```python
from build123d import *

# Parameters (mm, degrees)
CROQUIS1_W                         = 730
CROQUIS1_H                         = 400
BRIDA_BASE1_DEPTH                  = 2.9
BRIDA_DE_ARISTA1_STRIP_W           = 13.0732
BRIDA_DE_ARISTA1_STRIP_H           = 2.9
BRIDA_DE_ARISTA1_STRIP_CUT_DEPTH   = 730
BRIDA_DE_ARISTA1_STRIP_2_W         = 13.0732
BRIDA_DE_ARISTA1_STRIP_2_H         = 2.9
BRIDA_DE_ARISTA1_STRIP_CUT_2_DEPTH = 730
BRIDA_DE_ARISTA1_DEPTH             = 730
BRIDA_DE_ARISTA1_BEND_DEPTH        = 730
BRIDA_DE_ARISTA2_STRIP_W           = 13.0732
BRIDA_DE_ARISTA2_STRIP_H           = 2.9
BRIDA_DE_ARISTA2_STRIP_CUT_DEPTH   = 730
BRIDA_DE_ARISTA2_STRIP_2_W         = 13.0732
BRIDA_DE_ARISTA2_STRIP_2_H         = 2.9
BRIDA_DE_ARISTA2_STRIP_CUT_2_DEPTH = 730
BRIDA_DE_ARISTA2_DEPTH             = 730
BRIDA_DE_ARISTA2_BEND_DEPTH        = 730
CROQUIS18_W                        = 653.8
CROQUIS18_H                        = 36.3634
CORTAR_EXTRUIR1_DEPTH              = 4


# Sheet-metal steps are written as plain solids
with BuildPart() as part:
    # Croquis1 → Brida base1 (new body)
    with BuildSketch(Plane(origin=(0, 0, 0), x_dir=(1, 0, 0), z_dir=(0, 1, 0))):
        Rectangle(CROQUIS1_W, CROQUIS1_H)
    extrude(amount=-BRIDA_BASE1_DEPTH)

    # Brida de arista1 strip (across the edge) → Brida de arista1 strip cut (cut)
    with BuildSketch(Plane(origin=(365, 0, -200), x_dir=(0, 0, 1), z_dir=(-1, 0, 0))):
        with Locations((-2.9, -1.45)):
            Rectangle(BRIDA_DE_ARISTA1_STRIP_W, BRIDA_DE_ARISTA1_STRIP_H)
    extrude(amount=BRIDA_DE_ARISTA1_STRIP_CUT_DEPTH, mode=Mode.SUBTRACT)

    # Brida de arista1 strip 2 (across the edge) → Brida de arista1 strip cut 2 (cut)
    with BuildSketch(Plane(origin=(-365, 0, 200), x_dir=(0, 0, -1), z_dir=(1, 0, 0))):
        with Locations((-2.9, -1.45)):
            Rectangle(BRIDA_DE_ARISTA1_STRIP_2_W, BRIDA_DE_ARISTA1_STRIP_2_H)
    extrude(amount=BRIDA_DE_ARISTA1_STRIP_CUT_2_DEPTH, mode=Mode.SUBTRACT)

    # Brida de arista1 section (across the edge) → Brida de arista1 (add)
    with BuildSketch(Plane(origin=(365, 0, -200), x_dir=(0, 0, 1), z_dir=(-1, 0, 0))):
        with BuildLine():
            Line((0, 0.7366), (0, 272.1))
            Line((0, 272.1), (2.9, 272.1))
            Line((2.9, 272.1), (2.9, 0.7366))
            ThreePointArc((2.9, 0.7366), (3.115745145, 0.215745145), (3.6366, 0))
            Line((3.6366, 0), (3.6366, -2.9))
            ThreePointArc((3.6366, -2.9), (1.06513548, -1.83486452), (0, 0.7366))
        make_face()
    extrude(amount=BRIDA_DE_ARISTA1_DEPTH)

    # Brida de arista1 section 2 (across the edge) → Brida de arista1 bend (add)
    with BuildSketch(Plane(origin=(-365, 0, 200), x_dir=(0, 0, -1), z_dir=(1, 0, 0))):
        with BuildLine():
            Line((0, 0.7366), (0, 272.1))
            Line((0, 272.1), (2.9, 272.1))
            Line((2.9, 272.1), (2.9, 0.7366))
            ThreePointArc((2.9, 0.7366), (3.115745145, 0.215745145), (3.6366, 0))
            Line((3.6366, 0), (3.6366, -2.9))
            ThreePointArc((3.6366, -2.9), (1.06513548, -1.83486452), (0, 0.7366))
        make_face()
    extrude(amount=BRIDA_DE_ARISTA1_BEND_DEPTH)

    # Brida de arista2 strip (across the edge) → Brida de arista2 strip cut (cut)
    with BuildSketch(Plane(origin=(365, 272.1, -197.1), x_dir=(0, -1, 0), z_dir=(-1, 0, 0))):
        with Locations((-2.9, -1.45)):
            Rectangle(BRIDA_DE_ARISTA2_STRIP_W, BRIDA_DE_ARISTA2_STRIP_H)
    extrude(amount=BRIDA_DE_ARISTA2_STRIP_CUT_DEPTH, mode=Mode.SUBTRACT)

    # Brida de arista2 strip 2 (across the edge) → Brida de arista2 strip cut 2 (cut)
    with BuildSketch(Plane(origin=(-365, 272.1, 197.1), x_dir=(0, -1, 0), z_dir=(1, 0, 0))):
        with Locations((-2.9, -1.45)):
            Rectangle(BRIDA_DE_ARISTA2_STRIP_2_W, BRIDA_DE_ARISTA2_STRIP_2_H)
    extrude(amount=BRIDA_DE_ARISTA2_STRIP_CUT_2_DEPTH, mode=Mode.SUBTRACT)

    # Brida de arista2 section (across the edge) → Brida de arista2 (add)
    with BuildSketch(Plane(origin=(365, 272.1, -197.1), x_dir=(0, -1, 0), z_dir=(-1, 0, 0))):
        with BuildLine():
            Line((0, 0.7366), (0, 37.1))
            Line((0, 37.1), (2.9, 37.1))
            Line((2.9, 37.1), (2.9, 0.7366))
            ThreePointArc((2.9, 0.7366), (3.115745145, 0.215745145), (3.6366, 0))
            Line((3.6366, 0), (3.6366, -2.9))
            ThreePointArc((3.6366, -2.9), (1.06513548, -1.83486452), (0, 0.7366))
        make_face()
    extrude(amount=BRIDA_DE_ARISTA2_DEPTH)

    # Brida de arista2 section 2 (across the edge) → Brida de arista2 bend (add)
    with BuildSketch(Plane(origin=(-365, 272.1, 197.1), x_dir=(0, -1, 0), z_dir=(1, 0, 0))):
        with BuildLine():
            Line((0, 0.7366), (0, 37.1))
            Line((0, 37.1), (2.9, 37.1))
            Line((2.9, 37.1), (2.9, 0.7366))
            ThreePointArc((2.9, 0.7366), (3.115745145, 0.215745145), (3.6366, 0))
            Line((3.6366, 0), (3.6366, -2.9))
            ThreePointArc((3.6366, -2.9), (1.06513548, -1.83486452), (0, 0.7366))
        make_face()
    extrude(amount=BRIDA_DE_ARISTA2_BEND_DEPTH)

    # Croquis18 → Cortar-Extruir1 (cut)
    with BuildSketch(Plane(origin=(0, 272.1, 0), x_dir=(1, 0, 0), z_dir=(0, 1, 0))):
        with Locations((0, -178.1817)):
            Rectangle(CROQUIS18_W, CROQUIS18_H)
        with Locations((0, 178.1817)):
            Rectangle(CROQUIS18_W, CROQUIS18_H)
    extrude(amount=-CORTAR_EXTRUIR1_DEPTH, mode=Mode.SUBTRACT)


solid = part.part
```
CAD build for the part. Positions are in the model's coordinates, mm. A direction names the side the tool comes from. Coordinates: 2 decimals unless noted, no trailing zeros. Write each loop counter-clockwise with the first axis right and the second up, starting at its lowest first coordinate (ties: lowest second). Pieces come first, ordered by that corner, then holes. Notation, with made-up numbers: (-38.75, 87.25) -> (-34.75, 87.25) arc R36 ccw to (-34.75, 123.25) -> close; hole circle Ø2 at (10, 26). An arc over 180 degrees is marked (long way). Return JSON: item names as keys, results as strings. Group by question number.
Q1. Drill centre lines: line 1 (Z direction, x = -223.5, y = 226.5); line 2 (Y direction, x = 2, z = 19). Where is each one in solid material? Low to high.
Q2. Flat gauge pins, fed straight in: pin 1 (2.5 mm diameter, centred on x = 346, y = 270.5, fed in from -Z); pin 2 (3 mm diameter, centred on x = -353, y = 271, fed in from -Z); pin 3 (0.9 mm diameter, centred on x = -336.5, y = 270.5, fed in from +Z). Where does each tip first touch, or does it go through?
Q3. Cut at B-B, the plane x = -58. Give the cut face in (y, z), then the cut area to 3 significant figures.
Q4. Pull direction Y, two halves, no side cores. Call faces 3 (the face through (-5, -2.9, -3)), 4 (the face through (-346, 272.1, 178)), 5 (the face through (5, 136, -197.1)), 6 (the face through (-346, 269.2, -178)): released by +Y, released by -Y, zero draft, split by the parting line, or undercut.
Q5. Cut at A-A, the plane y = 208. Give the cut face in (x, z).
Q6. Cut at C-C, the plane z = -49.5. Give the cut face in (x, y).
Q7. Which spindle directions (+Z, -Z, +X, -X, +Y, -Y) get a long thin tool onto all of the face, cutting with end or side? Do faces 1 (the face through (346, 272.1, -178)), 2 (the face through (346, 269.2, -178)). Say none if no direction does.
Returned:
{
 "1": {"line 1": "z = -200 to -197.1, 197.1 to 200", "line 2": "y = -2.9 to 0"},
 "2": {"pin 1": "stops at z = -199.91", "pin 2": "stops at z = -199.85", "pin 3": "stops at z = 199.64"},
 "3": {"outline": "(-2.9, -196.36) arc R3.64 ccw to (0.74, -200) -> (268.46, -200) arc R3.64 ccw to (272.1, -196.36) -> (269.2, -196.36) arc R0.74 cw to (268.46, -197.1) -> (0.74, -197.1) arc R0.74 cw to (0, -196.36) -> (0, 196.36) arc R0.74 cw to (0.74, 197.1) -> (268.46, 197.1) arc R0.74 cw to (269.2, 196.36) -> (272.1, 196.36) arc R3.64 ccw to (268.46, 200) -> (0.74, 200) arc R3.64 ccw to (-2.9, 196.36) -> close", "area": "2,730 mm2"},
 "4": {"face 3": "released by -Y", "face 4": "released by +Y", "face 5": "undercut", "face 6": "undercut"},
 "5": {"outline": "(-365, -200) -> (365, -200) -> (365, -197.1) -> (-365, -197.1) -> close; (-365, 197.1) -> (365, 197.1) -> (365, 200) -> (-365, 200) -> close"},
 "6": {"outline": "(-365, -2.9) -> (365, -2.9) -> (365, 0) -> (-365, 0) -> close"},
 "7": {"face 1": "+Z, -Z, +X, -X, +Y", "face 2": "+X, -X"}
}
